Part model, mm, in its own coordinate system. A direction names the side the tool comes from. Round coordinates to 2 decimals unless told otherwise and drop trailing zeros. Order: outer loops, then holes, each group sorted by start corner. A loop starts at its lowest first (then second) coordinate and runs counter-clockwise, first axis right, second up. Notation, with made-up numbers: (7, 10) - (11, 10) arc R15 ccw to (11, 28) - close; hole circle Ø8 at (55, 39.25). An arc over 180 degrees is marked (long way). Answer as a JSON object with one key per item and string values.
```python
from build123d import *

# Parameters (mm, degrees)
EXTRUDE_2_DEPTH     = 3.4
CUT_EXTRUDE_3_DEPTH = 1


with BuildPart() as part:
    # 스케치7 → 보스-돌출2 (new body)
    with BuildSketch(Plane.XY):
        Polygon((-33.25966317, -13.776603565), (-13.776603565, -33.25966317), (13.776603565, -33.25966317), (33.25966317, -13.776603565), (33.25966317, 13.776603565), (13.776603565, 33.25966317), (-13.776603565, 33.25966317), (-33.25966317, 13.776603565), align=None)
        Polygon((-13.27954729, -32.05966317), (13.27954729, -32.05966317), (32.05966317, -13.27954729), (32.05966317, 13.27954729), (13.27954729, 32.05966317), (-13.27954729, 32.05966317), (-32.05966317, 13.27954729), (-32.05966317, -13.27954729), align=None, mode=Mode.SUBTRACT)
        Polygon((-32.05966317, -13.27954729), (-13.27954729, -32.05966317), (13.27954729, -32.05966317), (32.05966317, -13.27954729), (32.05966317, 13.27954729), (13.27954729, 32.05966317), (-13.27954729, 32.05966317), (-32.05966317, 13.27954729), align=None)
        Polygon((-12.782491015, -30.85966317), (12.782491015, -30.85966317), (30.85966317, -12.782491015), (30.85966317, 12.782491015), (12.782491015, 30.85966317), (-12.782491015, 30.85966317), (-30.85966317, 12.782491015), (-30.85966317, -12.782491015), align=None, mode=Mode.SUBTRACT)
        Polygon((-30.85966317, -12.782491015), (-12.782491015, -30.85966317), (12.782491015, -30.85966317), (30.85966317, -12.782491015), (30.85966317, 12.782491015), (12.782491015, 30.85966317), (-12.782491015, 30.85966317), (-30.85966317, 12.782491015), align=None)
        Polygon((-12.285434741, -29.65966317), (12.285434741, -29.65966317), (29.65966317, -12.285434741), (29.65966317, 12.285434741), (12.285434741, 29.65966317), (-12.285434741, 29.65966317), (-29.65966317, 12.285434741), (-29.65966317, -12.285434741), align=None, mode=Mode.SUBTRACT)
    extrude(amount=-EXTRUDE_2_DEPTH)

    # 스케치9 → 컷-돌출3 (cut)
    with BuildSketch(Plane.XY):
        Polygon((13.27954729, -32.05966317), (32.05966317, -13.27954729), (32.05966317, 13.27954729), (13.27954729, 32.05966317), (-13.27954729, 32.05966317), (-32.05966317, 13.27954729), (-32.05966317, -13.27954729), (-13.27954729, -32.05966317), align=None)
        Polygon((12.782491015, -30.85966317), (30.85966317, -12.782491015), (30.85966317, 12.782491015), (12.782491015, 30.85966317), (-12.782491015, 30.85966317), (-30.85966317, 12.782491015), (-30.85966317, -12.782491015), (-12.782491015, -30.85966317), align=None, mode=Mode.SUBTRACT)
    cut_extrude_3 = extrude(amount=-CUT_EXTRUDE_3_DEPTH, mode=Mode.SUBTRACT)

    # 대칭 복사4: 컷-돌출3 across plane
    add(cut_extrude_3.mirror(Plane.XY.offset(-1.7)), mode=Mode.SUBTRACT)


solid = part.part
```
Item 1: Probe L1, parallel to Y at x = 9, z = -0.2; L2, parallel to Y at x = -23.5, z = -0.6; L3, parallel to X at y = 6, z = -1.15. List the from-to ranges inside material, lowest first. Write a range as from..to.
Taken from the geometry:
{"L1": "-33.26..-32.06, -30.86..-29.66, 29.66..30.86, 32.06..33.26", "L2": "-23.54..-21.84, -20.14..-18.45, 18.45..20.14, 21.84..23.54", "L3": "-33.26..-29.66, 29.66..33.26"}
Item 2: Two-plate mould, pull along X, no slides. Class faces 5 (the flat face through (23.382, -23.655, -1.676)), 6 (the flat face through (-21.69, 21.95, -2.91)), 7 (the flat face through (0, 33.26, -2)): pulls with the +X half, pulls with the -X half, needs draft (parallel to the pull), parting line crosses it, or undercut.
Taken from the geometry:
{"face 5": "pulls with the +X half", "face 6": "undercut", "face 7": "needs draft"}
Item 3: Tool access for faces 1 (the flat face through (-21.95, -21.69, -2.91)), 2 (the flat face through (-22.8, -22.54, -0.49)), 3 (the flat face through (-33.26, 0, -2)), 4 (the flat face through (0, -29.66, -2)): list every direction of +Z, -Z, +X, -X, +Y, -Y with a clear straight run to the whole face (end or side of a thin tool).
Taken from the geometry:
{"face 1": "-Z", "face 2": "+Z", "face 3": "+Z, -Z, -X, +Y, -Y", "face 4": "+Z, -Z"}
Item 4: Cut at A-A (y = 11). Write the cut outline in (x, z), plus the area to 3 significant figures.
Taken from the geometry:
{"outline": "(-33.26, -3.4) - (-32.06, -3.4) - (-32.06, -2.4) - (-30.86, -2.4) - (-30.86, -3.4) - (-29.66, -3.4) - (-29.66, 0) - (-30.86, 0) - (-30.86, -1) - (-32.06, -1) - (-32.06, 0) - (-33.26, 0) - close; (29.66, -3.4) - (30.86, -3.4) - (30.86, -2.4) - (32.06, -2.4) - (32.06, -3.4) - (33.26, -3.4) - (33.26, 0) - (32.06, 0) - (32.06, -1) - (30.86, -1) - (30.86, 0) - (29.66, 0) - close", "area": "19.7 mm2"}
